from build123d import *

# Parameters (mm, degrees)
SKETCH1_W           = 30
SKETCH1_H           = 20
BOSS_EXTRUDE1_DEPTH = 15
SKETCH1_3_W         = 25
SKETCH1_3_H         = 15
BOSS_EXTRUDE2_DEPTH = 40


with BuildPart() as part:
    # Sketch1 → Boss-Extrude1 (new body)
    with BuildSketch(Plane(origin=(0, 0, 0), x_dir=(1, 0, 0), z_dir=(0, 1, 0))):
        Polygon((-25, -15), (-25, -30), (25, -30), (25, -15), (50, -15), (50, 15), (25, 15), (25, 30), (-25, 30), (-25, 15), (-50, 15), (-50, -15), align=None)
        Rectangle(SKETCH1_W, SKETCH1_H, mode=Mode.SUBTRACT)
    extrude(amount=BOSS_EXTRUDE1_DEPTH)

    # Sketch1<3> → Boss-Extrude2 (add)
    with BuildSketch(Plane(origin=(0, 0, 0), x_dir=(1, 0, 0), z_dir=(0, 1, 0))):
        with Locations((-37.5, 22.5)):
            Rectangle(SKETCH1_3_W, SKETCH1_3_H)
        with Locations((37.5, -22.5)):
            Rectangle(SKETCH1_3_W, SKETCH1_3_H)
    extrude(amount=BOSS_EXTRUDE2_DEPTH)


solid = part.part
Could you check a few things on this model? Use its own coordinates, in mm. A direction names the side the tool comes from. Coordinates: 2 decimals unless noted, no trailing zeros. Write each loop counter-clockwise with the first axis right and the second up, starting at its lowest first coordinate (ties: lowest second). Pieces come first, ordered by that corner, then holes. Notation, with made-up numbers: (28, -40) - (60, -40) arc R18 cw to (60, -16) - close; hole circle Ø6 at (5, 41.5). An arc over 180 degrees is marked (long way). Write item = value, one per line.
1) For faces 5 (the flat face through (38, 7, -15)), 6 (the flat face through (25, 27, 23)), 7 (the flat face through (37, 27, 15)), 8 (the flat face through (-38, 7, 15)), which set-ups out of +Z, -Z, +X, -X, +Y, -Y let a thin tool reach every point of the face, with its end or its side?
Result set:
face_5 = -Z, +X, +Y, -Y
face_6 = +Z, -Z, -X, +Y
face_7 = -Z, +X, -X, +Y
face_8 = +Z, -X, +Y, -Y
2) Suppose I cut it at D-D on z = -24. Please give me the cut outline in (x, y).
Result set:
outline = (-50, 0) - (25, 0) - (25, 15) - (-25, 15) - (-25, 40) - (-50, 40) - close
3) Please list where these lines run through material, in increasing order: line 1 (Z direction, x = -8, y = 7); line 2 (Y direction, x = -41, z = 12.5); line 3 (Z direction, x = 33, y = 34). Write a range as [from, to].
Result set:
line_1 = [-30, -10], [10, 30]
line_2 = [0, 15]
line_3 = [15, 30]
4) Will these pins go through, and if not, where does the flat tip stop? pin 1 Ø4.5 at (x, y) = (33, 11) entering from -Z; pin 2 Ø4.5 at (y, z) = (27.5, 23.5) entering from -X; pin 3 Ø7.5 at (x, y) = (-41.5, 5) entering from +Z.
Result set:
pin_1 = -15
pin_2 = 25
pin_3 = 15
5) Suppose I cut it at B-B on z = -6. Please give me the cut outline in (x, y), plus the area to 3 significant figures.
Result set:
outline = (-50, 0) - (-15, 0) - (-15, 15) - (-50, 15) - close; (15, 0) - (50, 0) - (50, 15) - (15, 15) - close
area = 1,050 mm2
6) Suppose I cut it at C-C on y = 28. Please give me the cut outline in (x, z), plus the area to 3 significant figures.
Result set:
outline = (-50, -30) - (-25, -30) - (-25, -15) - (-50, -15) - close; (25, 15) - (50, 15) - (50, 30) - (25, 30) - close
area = 750 mm2
7) Suppose I cut it at A-A on y = 3. Please give me the cut outline in (x, z).
Result set:
outline = (-50, -30) - (25, -30) - (25, -15) - (50, -15) - (50, 30) - (-25, 30) - (-25, 15) - (-50, 15) - close; hole (-15, -10) - (15, -10) - (15, 10) - (-15, 10) - close
8) We'd pull the mould along Z, two halves only. Please class faces 1 (the flat face through (-15, 7, 0)), 2 (the flat face through (-25, 7, 22)), 3 (the flat face through (0, 7, 10)), 4 (the flat face through (-38, 27, -15)): +Z half, -Z half, draft (parallel to the pull), parting line (faces both ways), or undercut.
Result set:
face_1 = undercut
face_2 = draft
face_3 = undercut
face_4 = +Z half
